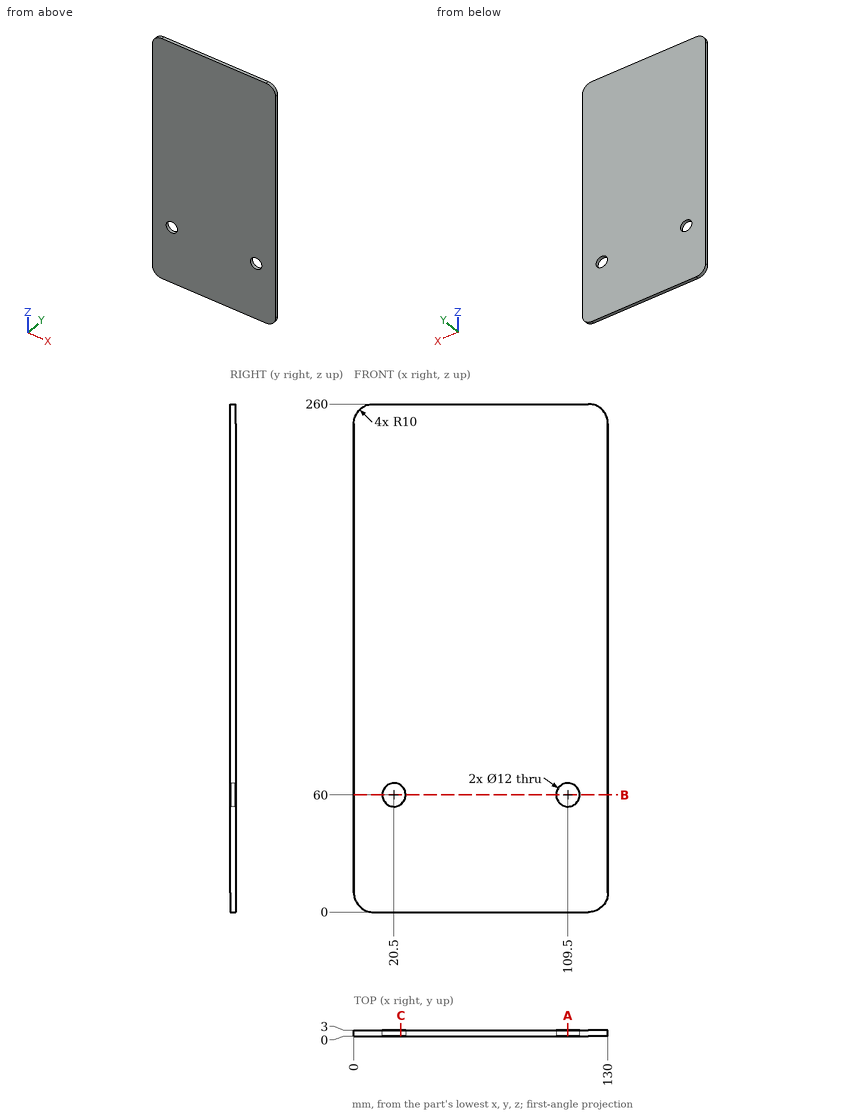
Part print with two shaded views. Sizes in mm from the minimum x, y, z corner. Round coordinates to 2 decimals unless told otherwise and drop trailing zeros. Loops run counter-clockwise (first coordinate to the right, second up) from the corner with the lowest first, then second, coordinate; pieces in that order, holes last.
Item 1: Saw through at A-A (x = 109.5). List the corners of the cut face in (y, z).
Item 2: Drill centre lines: line 1 along Z through (x, y) = (20.5, 1.2); line 2 along Z through (x, y) = (21.5, 2); line 3 along Z through (x, y) = (5, 2). Where is each one in solid material? Low to high.
Item 3: Saw through at C-C (x = 24). List the corners of the cut face in (y, z).
Item 4: Saw through at B-B (z = 60). List the corners of the cut face in (x, y), then the cut area to 3 significant figures.
Item 5: Pin check, flat tip, straight feed: P1, Ø19, axis at x = 20.5, z = 60, coming from the -Y side. Stop position of the tip, or through.
Worked answers:
1. outline: (0, 0) - (3, 0) - (3, 54) - (0, 54) - close; (0, 66) - (3, 66) - (3, 260) - (0, 260) - close
2. line 1: z = 0 to 54, 66 to 260
2. line 2: z = 0 to 54.08, 65.92 to 260
2. line 3: z = 1.34 to 258.66
3. outline: (0, 0) - (3, 0) - (3, 55.13) - (0, 55.13) - close; (0, 64.87) - (3, 64.87) - (3, 260) - (0, 260) - close
4. outline: (0, 0) - (14.5, 0) - (14.5, 3) - (0, 3) - close; (26.5, 0) - (103.5, 0) - (103.5, 3) - (26.5, 3) - close; (115.5, 0) - (130, 0) - (130, 3) - (115.5, 3) - close
4. area: 318 mm2
5. P1: stops at y = 0
